Autodesk Inventor part; units mm, degrees
ref_plane "YZ Plane" through (0, 0, 0) normal (1, 0, 0) x (0, 1, 0)
ref_plane "XZ Plane" through (0, 0, 0) normal (0, 1, 0) x (-1, 0, 0)
ref_plane "XY Plane" through (0, 0, 0) normal (0, 0, 1) x (1, 0, 0)
sketch "Sketch1" plane through (0, 0, 0) normal (0, 1, 0) x (-1, 0, 0)
  circle A0 centre (0, 0) radius 50 construction
  circle A1 centre (50, 0) radius 4
  line L0 (0, 0) -> (43.3013, -25) construction
  line L1 (0, 0) -> (50, 0) construction
  circle A2 centre (43.3013, -25) radius 4
  circle A3 centre (43.3013, 25) radius 4
  circle A4 centre (0, 50) radius 4
  circle A5 centre (-43.3013, 25) radius 4
  circle A6 centre (-43.3013, -25) radius 4
  circle A7 centre (0, -50) radius 4
  line L2 (25, 55.25) -> (-25, 55.25)
  arc A8 (-53.8355, 31.903) -> (-62.5784, 0) centre (0, 0) ccw
  arc A9 (62.5784, 0) -> (53.8355, 31.903) centre (0, 0) ccw
  line L3 (0, 55.25) -> (40, 55.25)
  line L4 (0, 55.25) -> (-40, 55.25)
  line L5 (40, 55.25) -> (53.8355, 31.903)
  line L6 (-40, 55.25) -> (-53.8355, 31.903)
  line L7 (62.5784, 0) -> (-62.5784, 0) construction
  arc A10 (-62.5784, 0) -> (-53.8355, -31.903) centre (0, 0) ccw
  arc A11 (53.8355, -31.903) -> (62.5784, 0) centre (0, 0) ccw
  line L8 (0, -55.25) -> (40, -55.25)
  line L9 (0, -55.25) -> (-40, -55.25)
  line L10 (40, -55.25) -> (53.8355, -31.903)
  line L11 (-40, -55.25) -> (-53.8355, -31.903)
  point P0 (-25, 55.25)
  dimension "d1" = 100
  dimension "d2" = 8
  dimension "d3" = 30
  dimension "d4" = 8
  dimension "d7" = 360
  dimension "d35" = 40
  dimension "d36" = 40
  dimension "d49" = 110.5
extrude "Extrusion1" add sketch "Sketch1" along normal blind 15
sketch "Sketch4" plane through (-40, 0, 55.25) normal (0, 0, 1) x (1, 0, 0)
  line L0 (40, 200) -> (40, 184) construction
  line L1 (40, 184) -> (40, 180) construction
  circle A0 centre (40, 180) radius 4
  line L2 (40, 180) -> (40, 150) construction
  circle A1 centre (40, 150) radius 4
  arc A2 (59.9595, 181.2724) -> (20.0405, 181.2724) centre (40, 180) ccw
  line L3 (0, 0) -> (0, 15)
  line L4 (0, 15) -> (0, 0)
  line L5 (80, 0) -> (80, 15)
  line L6 (0, 0) -> (80, 0)
  line L7 (80, 0) -> (80, 15)
  line L8 (40, 0) -> (40, 15) construction
  line L9 (40, 146) -> (40, 200) construction
  line L10 (20.0405, 181.2724) -> (20.0405, 131.2724)
  line L11 (0, 15) -> (0, 35)
  line L12 (59.9595, 181.2724) -> (59.9595, 128.6983)
  line L13 (0, 15) -> (80, 15)
  line L14 (80, 15) -> (80, 35)
  arc A3 (0, 35) -> (20.0405, 131.2724) centre (-221.2208, 131.2724) ccw
  arc A4 (59.9595, 128.6983) -> (80, 35) centre (289.0202, 128.6983) ccw
  dimension "d42" = 8
  dimension "d37" = 200
  dimension "d38" = 16
  dimension "d39" = 4
  dimension "d40" = 8
  dimension "d41" = 30
  dimension "d50" = 50
  dimension "d51" = 20
  dimension "d52" = 20
extrude "Extrusion3" add sketch "Sketch4" along normal blind 15
mirror "Mirror2" about plane through (0, 0, 0) normal (0, 0, 1) of "Extrusion3"
properties part number "MOUNTING-COUPLE"
Here's how the part is built. I have some questions about the finished solid (model axes, mm). A direction names the side the tool comes from. Round coordinates to 2 decimals unless told otherwise and drop trailing zeros. Order: outer loops, then holes, each group sorted by start corner. A loop starts at its lowest first (then second) coordinate and runs counter-clockwise, first axis right, second up. Notation, with made-up numbers: M 63.5,83.5 L 111.5,83.5 A8 ccw 111.5,95.5 Z; hole C 14.5,40 d8. An arc over 180 degrees is marked long. Use CSV: the item, a comma, the result in double quotes.
1) I'm going to push flat-ended pins straight in: P1, Ø13, axis at x = -50, z = 0, coming from the -Y side; P2, Ø12, axis at y = 20.5, z = -64, coming from the -X side; P3, Ø7.5, axis at y = 9.5, z = -64.5, coming from the +X side; P4, Ø12, axis at y = 146, z = 61.5, coming from the +X side. Where does each tip first touch, or does it pass through?
Taken from the geometry:
P1,"y = 0"
P2,"x = -40"
P3,"x = 40"
P4,"x = 19.96"
2) I need wall thicknesses on line 1 along Z through (x, y) = (5, 32.5); line 2 along Y through (x, z) = (-3, 61.5); line 3 along X through (y, z) = (9.5, 61). Which ranges of each line are inside material? Lowest first, please. Write a range as [from, to].
Taken from the geometry:
line 1,"[-70.25, -55.25], [55.25, 70.25]"
line 2,"[0, 147.35], [152.65, 177.35], [182.65, 199.77]"
line 3,"[-40, 40]"
3) I want a section at D-D (x = 45). List the corners of the cut face in (y, z) for me.
Taken from the geometry:
outline,"M 0,-46.81 L 15,-46.81 L 15,-28.62 L 0,-28.62 Z; M 0,-21.38 L 15,-21.38 L 15,21.38 L 0,21.38 Z; M 0,28.62 L 15,28.62 L 15,46.81 L 0,46.81 Z"
4) I want a section at A-A (y = 173). List the corners of the cut face in (x, z) for me.
Taken from the geometry:
outline,"M -19.96,-70.25 L 19.96,-70.25 L 19.96,-55.25 L -19.96,-55.25 Z; M -19.96,55.25 L 19.96,55.25 L 19.96,70.25 L -19.96,70.25 Z"
5) I want a section at B-B (x = 0). Count the separate pieces of the cut face and the enclosed holes in it, then the cut area to 3 significant figures.
Taken from the geometry:
separate pieces,"7"
enclosed holes,"0"
area,"6,940 mm^2"
6) On a 3-axis mill with a long thin cutter (end or side, diameter ignored), from which of +Z, -Z, +X, -X, +Y, -Y can I reach the whole of each face in a straight line? I mean faces 4 (the flat face through (46.82, 7.4, 43.74)), 5 (the flat face through (-40, 18, -63)), 6 (the flat face through (-19.96, 156, -63)). Say none if no direction works.
Taken from the geometry:
face 4,"+Z, +X, +Y, -Y"
face 5,"-Z, -X, +Y, -Y"
face 6,"+Z, -Z, -X, +Y"
7) I want a section at C-C (z = 25). List the corners of the cut face in (x, y) for me, then the cut area to 3 significant figures.
Taken from the geometry:
outline,"M -57.37,0 L -47.3,0 L -47.3,15 L -57.37,15 Z; M -39.3,0 L 39.3,0 L 39.3,15 L -39.3,15 Z; M 47.3,0 L 57.37,0 L 57.37,15 L 47.3,15 Z"
area,"1,480 mm^2"
8) If we mould it in two halves opening along Y, with no side actions, what happens to faces 1 (the flat face through (1, 88, -55.25)), 2 (the cylindrical face through (0, 200, -63)), 3 (the cylindrical face through (-0.521, 183.966, -62.645))? For each: pulls with the +Y half, pulls with the -Y half, needs draft (parallel to the pull), parting line crosses it, or undercut.
Taken from the geometry:
face 1,"needs draft"
face 2,"pulls with the +Y half"
face 3,"undercut"
